Could you check a few things on this model? Use its own coordinates, in mm. A direction names the side the tool comes from. Give positions to 0.01 mm unless a question says otherwise; leave off trailing zeros. Loops run counter-clockwise (first coordinate to the right, second up) from the corner with the lowest first, then second, coordinate; pieces in that order, holes last. Notation, with made-up numbers: (27.25, -29) - (57.25, -29) arc R6 ccw to (57.25, -18) - close; hole circle Ø2 at (3, 76.5). An arc over 180 degrees is marked (long way). Write each question's results on one line, items separated by ' | '. Start each with the question number.
1) I want a section at A-A, the plane x = 0. Write out the boundary of the cut face in (y, z).
2) If I drill on probe 1 along X at (y, z) = (-45.5, 0); probe 2 along Z at (x, y) = (0, -24); probe 3 along Z at (x, y) = (0, -47), over which ranges is the centre line in solid material (lowest first)? Write a range as [from, to].
3) I want a section at C-C, the plane z = 0. Write out the boundary of the cut face in (x, y), and give its area (3 significant figures).
4) If we mould it in two halves opening along Z, with no side actions, what happens to faces 1 (the face through (-136, -73.406, 0)), 2 (the face through (0, -25.947, 0)), 3 (the face through (-126, -36, -23.241))? For each: +Z half, -Z half, draft (parallel to the pull), parting line (faces both ways), or undercut.
5) I want a section at B-B, the plane y = -60. Write out the boundary of the cut face in (x, z), and give its area (3 significant figures).
6) On a 3-axis mill with a long thin cutter (end or side, diameter ignored), from which of +Z, -Z, +X, -X, +Y, -Y can I reach the whole of each face in a straight line? I mean faces 4 (the face through (-261, -30, -12.7)), 5 (the face through (-123, -36, 23.241)), 6 (the face through (25.39, -36.19, -0.71)), 7 (the face through (-260, -9.252, 0)), 8 (the face through (-293.452, -31, 0)). Say none if no direction works.
7) I want a section at D-D, the plane y = -15. Write out the boundary of the cut face in (x, z).
8) I'm going to push flat-ended pins straight in: pin 1 (8 mm diameter, centred on x = -64.5, y = -38, fed in from +Z); pin 2 (7.5 mm diameter, centred on x = -268, z = 4, fed in from -Y); pin 3 (8 mm diameter, centred on x = -8, y = -56, fed in from -Z). Where does each tip first touch, or does it pass through?
from build123d import *

# Parameters (mm, degrees)
F0_R     = 20.066
F1_DEPTH = 25.4
F2_DEPTH = 48.006
F3_W     = 1.0977562389
F3_H     = 41.91
F4_DEPTH = 12.7


with BuildPart() as f1:
    # F0 (on Front) → F1 (new body)
    with BuildSketch(Plane.XZ):
        with BuildLine():
            ThreePointArc((-10.2477275042, -23.241), (-25.4, 0), (-10.2477275042, 23.241))
            Line((-10.2477275042, 23.241), (-238.9725779709, 23.241))
            ThreePointArc((-238.9725779709, 23.241), (-231.493347745, 12.674084791), (-228.854, 0))
            ThreePointArc((-228.854, 0), (-231.493347745, -12.674084791), (-238.9725779709, -23.241))
            Line((-238.9725779709, -23.241), (-10.2477275042, -23.241))
        make_face()
        with BuildLine():
            ThreePointArc((-228.854, 0), (-231.493347745, 12.674084791), (-238.9725779709, 23.241))
            ThreePointArc((-238.9725779709, 23.241), (-292.354, 0), (-238.9725779709, -23.241))
            ThreePointArc((-238.9725779709, -23.241), (-231.493347745, -12.674084791), (-228.854, 0))
        make_face()
        with Locations((-260.604, 0)):
            Circle(F0_R, mode=Mode.SUBTRACT)
        with BuildLine():
            ThreePointArc((-10.2477275042, -23.241), (13.8720532257, -21.2773621322), (25.4, 0))
            ThreePointArc((25.4, 0), (13.8720532257, 21.2773621322), (-10.2477275042, 23.241))
            ThreePointArc((-10.2477275042, 23.241), (-25.4, 0), (-10.2477275042, -23.241))
        make_face()
        Circle(F0_R, mode=Mode.SUBTRACT)
    extrude(amount=F1_DEPTH)

    # F2 (add): a face of the model
    f2_faces = [f1.faces().sort_by_distance(p)[0] for p in [
        (-139.2710743105, -25.4, 0),
    ]]
    extrude(f2_faces, amount=F2_DEPTH)

    # F3 (on Top) → F4 (join, symmetric)
    with BuildSketch(Plane.XY):
        Polygon((-10.2477275042, 0), (-163.8780487135, 0), (-188.47713992, -9.2518740857), (-292.354, -9.2518740857), (-292.354, -51.1618740857), (-180.8564199804, -51.1618740857), (-113.8137692817, -25.9467083128), (-10.2477275042, -25.9467083128), align=None)
        Polygon((25.4, 0), (-10.2477275042, 0), (-10.2477275042, -25.9467083128), (25.713481009, -25.9467083128), (25.713481009, 0), align=None)
        with Locations((-292.9028781195, -30.2068740857)):
            Rectangle(F3_W, F3_H)
    extrude(amount=F4_DEPTH, both=True)


solid = f1.part
Answers:
1) outline: (-73.41, -25.4) - (0, -25.4) - (0, -20.07) - (-73.41, -20.07) - close; (-73.41, 20.07) - (0, 20.07) - (0, 25.4) - (-73.41, 25.4) - close; (-25.95, -12.7) - (0, -12.7) - (0, 12.7) - (-25.95, 12.7) - close
2) probe 1: x = [-293.45, -20.07], [20.07, 25.4] | probe 2: z = [-25.4, -20.07], [-12.7, 12.7], [20.07, 25.4] | probe 3: z = [-25.4, -20.07], [20.07, 25.4]
3) outline: (-293.45, -51.16) - (-292.35, -51.16) - (-292.35, -73.41) - (-280.67, -73.41) - (-280.67, -51.16) - (-240.54, -51.16) - (-240.54, -73.41) - (-20.07, -73.41) - (-20.07, -25.95) - (20.07, -25.95) - (20.07, -73.41) - (25.4, -73.41) - (25.4, -25.95) - (25.71, -25.95) - (25.71, 0) - (-240.54, 0) - (-240.54, -9.25) - (-280.67, -9.25) - (-280.67, 0) - (-292.35, 0) - (-292.35, -9.25) - (-293.45, -9.25) - close | area: 20,200 mm2
4) face 1: draft | face 2: undercut | face 3: -Z half
5) outline: (-238.97, -23.24) - (-10.25, -23.24) arc R25.4 ccw (long way) to (-10.25, 23.24) - (-238.97, 23.24) arc R31.75 ccw (long way) to start; hole circle Ø40.13 at (-260.6, 0); hole circle Ø40.13 at (0, 0) | area: 12,500 mm2
6) face 4: +Y, -Y | face 5: +Z, +Y, -Y | face 6: -Y | face 7: +Y | face 8: +Z, -Z, -X, +Y, -Y
7) outline: (-293.45, -12.7) - (-289.7, -12.7) arc R31.75 ccw to (-238.97, -23.24) - (-10.25, -23.24) arc R25.4 ccw to (22, -12.7) - (25.71, -12.7) - (25.71, 12.7) - (22, 12.7) arc R25.4 ccw to (-10.25, 23.24) - (-238.97, 23.24) arc R31.75 ccw to (-289.7, 12.7) - (-293.45, 12.7) - close; hole (-276.14, -12.7) arc R20.07 ccw to (-245.07, -12.7) - close; hole (-276.14, 12.7) - (-245.07, 12.7) arc R20.07 ccw to start; hole (-15.54, -12.7) arc R20.07 ccw to (15.54, -12.7) - close; hole (-15.54, 12.7) - (15.54, 12.7) arc R20.07 ccw to start
8) pin 1: stops at z = 23.24 | pin 2: stops at y = -51.16 | pin 3: stops at z = -25.08
